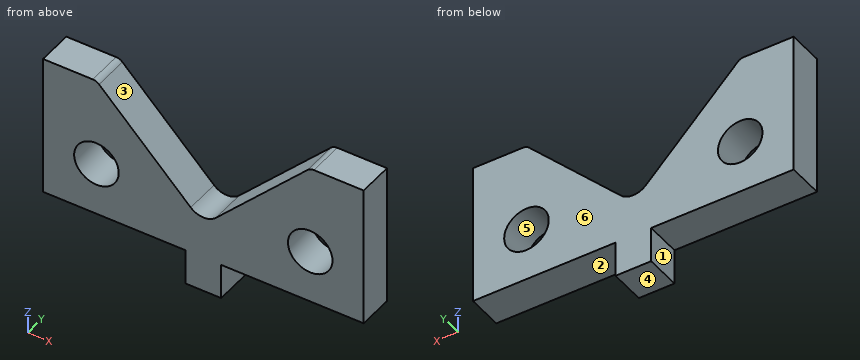
from build123d import *

# Parameters (mm, degrees)
F1_DEPTH = 12.7
F2_R     = 6.35
F3_R     = 3.175
F4_W     = 12.7
F4_H     = 12.7
F5_DEPTH = 12.7
F6_R     = 7.9375
F7_DEPTH = 25.4


with BuildPart() as f1:
    # F0 (on Front) → F1 (new body)
    with BuildSketch(Plane.XZ):
        Polygon((0, 50.8), (0, 0), (114.3, 0), (114.3, 50.8), (95.25, 50.8), (57.15, 12.7), (19.05, 50.8), align=None)
    extrude(amount=F1_DEPTH)

    # F2
    f2_edges = [f1.edges().sort_by_distance(p)[0] for p in [
        (57.15, -6.35, 12.7),
    ]]
    fillet(f2_edges, radius=F2_R)

    # F3
    f3_edges = [f1.edges().sort_by_distance(p)[0] for p in [
        (19.05, -6.35, 50.8),
        (95.25, -6.35, 50.8),
    ]]
    fillet(f3_edges, radius=F3_R)

    # F4 (on face) → F5 (join)
    with BuildSketch(Plane.XZ.offset(12.7)):
        with Locations((57.15, -6.35)):
            Rectangle(F4_W, F4_H)
    extrude(amount=-F5_DEPTH)

    # F6 (on face) → F7 (cut)
    with BuildSketch(Plane.XZ.offset(12.7)):
        with Locations((19.05, 19.05)):
            Circle(F6_R)
        with Locations((95.25, 19.05)):
            Circle(F6_R)
    extrude(amount=-F7_DEPTH, mode=Mode.SUBTRACT)


solid = f1.part
Model file for the job. Use its own axes, mm. Face numbers are marked on the shaded views. A direction names the side the tool comes from. Round coordinates to 2 decimals unless told otherwise and drop trailing zeros. Loops run counter-clockwise (first coordinate to the right, second up) from the corner with the lowest first, then second, coordinate; pieces in that order, holes last. Notation, with made-up numbers: (23.25, 61.5) -> (40.25, 61.5) arc R32 ccw to (40.25, 87.5) -> close; hole circle Ø6 at (81, 53.5). An arc over 180 degrees is marked (long way). Answer as CSV lines item,"result". Start each with the question number.
1) Slice it at C-C (y = -2). State how many separate pieces and enclosed holes the cut face has, plus the area to 3 significant figures.
2) Slice it at B-B (z = 19.05). List the corners of the cut face in (x, y).
3) Slice it at D-D (x = 100). List the corners of the cut face in (y, z).
4) Slice it at A-A (z = 38). List the corners of the cut face in (x, y), plus the area to 3 significant figures.
5) Mould opens along Z. For the marked faces 4, 5 and 6 say: +Z half, -Z half, draft (parallel to the pull), parting line (faces both ways), or undercut.
6) Pin check, flat tips, straight feed: P1, Ø4, axis at x = 77, y = -11.5, coming from the -Z side; P2, Ø14.5, axis at x = 95.25, z = 19.05, coming from the -Y side. Stop position of each tip, or through.
7) Probe line 1 along X through (y, z) = (-3.75, 26); line 2 along X through (y, z) = (-9.5, 35); line 3 along X through (y, z) = (-2, 46). List the from-to ranges inside material, lowest first.
8) Tool access for the marked faces 1, 2 and 3: list every direction of +Z, -Z, +X, -X, +Y, -Y with a clear straight run to the whole face (end or side of a thin tool).
Filled in:
1,separate pieces,"1"
1,enclosed holes,"2"
1,area,"4,130 mm2"
2,outline,"(0, -12.7) -> (11.11, -12.7) -> (11.11, 0) -> (0, 0) -> close; (26.99, -12.7) -> (50.8, -12.7) -> (50.8, 0) -> (26.99, 0) -> close; (63.5, -12.7) -> (87.31, -12.7) -> (87.31, 0) -> (63.5, 0) -> close; (103.19, -12.7) -> (114.3, -12.7) -> (114.3, 0) -> (103.19, 0) -> close"
3,outline,"(-12.7, 0) -> (0, 0) -> (0, 12.69) -> (-12.7, 12.69) -> close; (-12.7, 25.41) -> (0, 25.41) -> (0, 50.8) -> (-12.7, 50.8) -> close"
4,outline,"(0, -12.7) -> (31.85, -12.7) -> (31.85, 0) -> (0, 0) -> close; (82.45, -12.7) -> (114.3, -12.7) -> (114.3, 0) -> (82.45, 0) -> close"
4,area,"809 mm2"
5,face 4,"-Z half"
5,face 5,"undercut"
5,face 6,"draft"
6,P1,"stops at z = 0"
6,P2,"passes through"
7,line 1,"x = 0 to 15.22, 22.88 to 43.85, 70.45 to 91.42, 99.08 to 114.3"
7,line 2,"x = 0 to 34.85, 79.45 to 114.3"
7,line 3,"x = 0 to 23.85, 90.45 to 114.3"
8,face 1,"-Z, -X, +Y, -Y"
8,face 2,"-Z, +X, +Y, -Y"
8,face 3,"+Z, +Y, -Y"
